Geometry: see drawing. Coordinates: mm, zero at the bounding-box minimum. Give positions to 0.01 mm unless a question says otherwise; leave off trailing zeros. Loops run counter-clockwise (first coordinate to the right, second up) from the corner with the lowest first, then second, coordinate; pieces in that order, holes last. Notation, with made-up numbers: M -18.5,17.5 L 30.5,17.5 A24 ccw 30.5,46.5 Z; hole C -38.5,-8 d1. An arc over 180 degrees is marked long. Put each result on its own line as item: value.
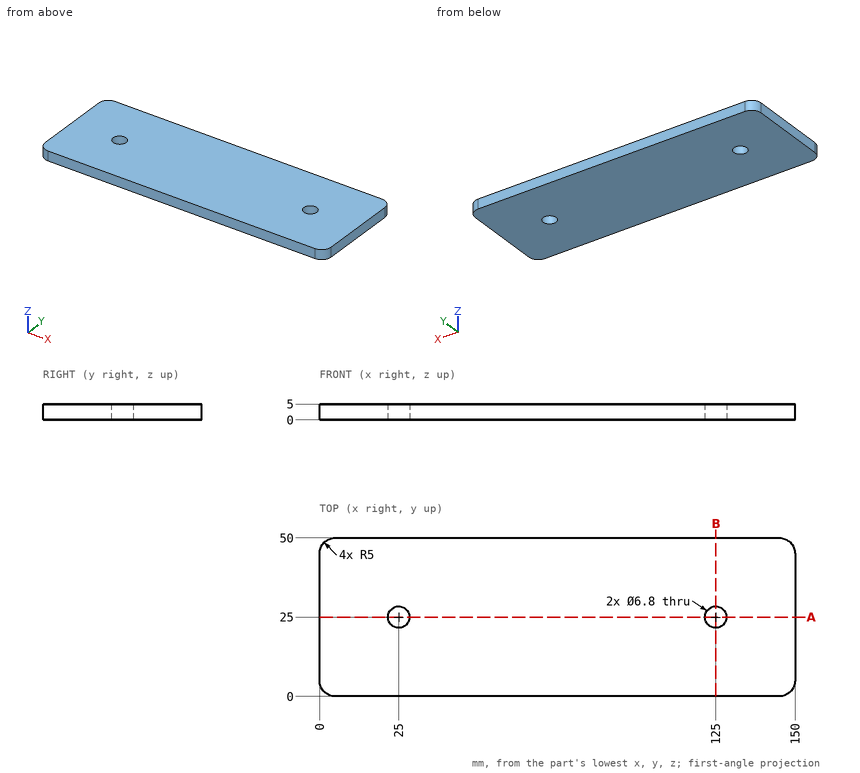
1. Contact query for a flat-ended pin moving along its axis: P1, Ø5.5, axis at x = 125, y = 25, coming from the -Z side. Output: stop coordinate, or through.
Found:
P1: through
2. Section query B-B (x = 125). Output: boundary loops of the cut face in (y, z), plus the area to 3 significant figures.
Found:
outline: M 0,0 L 21.6,0 L 21.6,5 L 0,5 Z; M 28.4,0 L 50,0 L 50,5 L 28.4,5 Z
area: 216 mm^2
3. Material intervals for line 1 (Y direction, x = 125, z = 4), sorted ascending. Write a range as from..to.
Found:
line 1: 0..21.6, 28.4..50
4. Section query A-A (y = 25). Output: boundary loops of the cut face in (x, z), plus the area to 3 significant figures.
Found:
outline: M 0,0 L 21.6,0 L 21.6,5 L 0,5 Z; M 28.4,0 L 121.6,0 L 121.6,5 L 28.4,5 Z; M 128.4,0 L 150,0 L 150,5 L 128.4,5 Z
area: 682 mm^2
